Can you work these out from the model? Positions are in its coordinate system, mm. A direction names the side the tool comes from. Round coordinates to 2 decimals unless told otherwise and drop trailing zeros. Loops run counter-clockwise (first coordinate to the right, second up) from the corner with the lowest first, then second, coordinate; pieces in that order, holes last. Notation, with made-up numbers: (-29, 35.5) -> (-11, 35.5) arc R18 cw to (-11, 55.5) -> close; hole circle Ø2 at (-39, 80). An arc over 180 degrees is marked (long way). Write item = value, one per line.
Autodesk Inventor part; units mm, degrees
ref_plane "YZ Plane" through (0, 0, 0) normal (1, 0, 0) x (0, 1, 0)
ref_plane "XZ Plane" through (0, 0, 0) normal (0, 1, 0) x (-1, 0, 0)
ref_plane "XY Plane" through (0, 0, 0) normal (0, 0, 1) x (1, 0, 0)
sketch "Sketch1" plane through (0, 0, 0) normal (0, 1, 0) x (-1, 0, 0)
  line L0 (0, 0) -> (105, 0)
  line L1 (105, 0) -> (105, 30)
  line L2 (105, 30) -> (0, 30)
  line L3 (0, 30) -> (0, 0)
  line L4 (105, 0) -> (65, 0)
  line L5 (65, 0) -> (65, 15)
  line L6 (65, 15) -> (105, 15)
  line L7 (105, 15) -> (105, 0)
  line L8 (0, 15) -> (15, 15)
  line L9 (15, 15) -> (45, 15)
  circle A0 centre (15, 15) radius 4
  circle A1 centre (45, 15) radius 7.5
  dimension "d0" = 105
  dimension "d1" = 30
  dimension "d2" = 40
  dimension "d3" = 15
  dimension "d4" = 15
  dimension "d5" = 30
  dimension "d6" = 8
  dimension "d7" = 15
extrude "Extrusion1" add sketch "Sketch1" along normal blind 55 contours L3 L2 L1 L6 L5 L0
sketch "Sketch2" plane through (-105, 0, 30) normal (0, 0, 1) x (1, 0, 0)
  line L0 (105, 55) -> (81, 55)
  line L1 (81, 55) -> (81, 15)
  line L2 (81, 15) -> (105, 15)
  line L3 (105, 15) -> (105, 55)
  dimension "d10" = 24
  dimension "d11" = 40
extrude "Extrusion2" cut sketch "Sketch2" against normal blind 55
sketch "Sketch3" plane through (-65, 0, 15) normal (0, 0, -1) x (-1, 0, 0)
  line L0 (40, 55) -> (0, 55)
  line L1 (0, 55) -> (0, 40)
  line L2 (0, 40) -> (40, 40)
  line L3 (40, 40) -> (40, 55)
  circle A0 centre (20, 20) radius 4
  point P0 (-65, 0)
  dimension "d15" = 15
  dimension "d16" = 8
extrude "Extrusion3" cut sketch "Sketch3" against normal blind 55
properties part number "X_Top_PullySide_V2" material "Birch"
1. Suppose I cut it at D-D, the plane z = 17.5. List the corners of the cut face in (x, y) for me.
Entries:
outline = (-105, 0) -> (-52.07, 0) -> (-52.07, 55) -> (-65, 55) -> (-65, 40) -> (-105, 40) -> close; (-37.93, 0) -> (-18.12, 0) -> (-18.12, 15) -> (-24, 15) -> (-24, 55) -> (-37.93, 55) -> close; (-11.88, 0) -> (0, 0) -> (0, 15) -> (-11.88, 15) -> close; hole circle Ø8 at (-85, 20)
2. For faces 4 (the cylindrical face through (-82.05, 22.7, 22.4)), 5 (the flat face through (-85, 40, 22)), 6 (the flat face through (-10, 15, 15)), 7 (the cylindrical face through (-52.154, 27.115, 12.747)), 8 (the flat face through (-80, 20, 15)), which set-ups out of +Z, -Z, +X, -X, +Y, -Y let a thin tool reach every point of the face, with its end or its side?
Entries:
face_4 = +Z, -Z
face_5 = +Z, -Z, -X, +Y
face_6 = +Z, -Z, +X, +Y
face_7 = +Y, -Y
face_8 = -Z, -X, +Y, -Y
3. I'm going to push flat-ended pins straight in: pin 1 (4 mm diameter, centred on y = 15, z = 17.5, fed in from +X); pin 2 (9 mm diameter, centred on y = 38, z = 19.5, fed in from +X); pin 3 (7.5 mm diameter, centred on x = -87.5, z = 24, fed in from +Y). Where does each tip first touch, or does it pass through?
Entries:
pin_1 = 0
pin_2 = -24
pin_3 = 40
4. We'd pull the mould along Z, two halves only. Please class faces 1 (the flat face through (-39, 27, 0)), 2 (the cylindrical face through (-11, 7, 15)), 3 (the flat face through (-52, 0, 19)): released by +Z, released by -Z, zero draft, split by the parting line, or undercut.
Entries:
face_1 = released by -Z
face_2 = undercut
face_3 = zero draft
5. Suppose I cut it at C-C, the plane y = 20. List the corners of the cut face in (x, z) for me.
Entries:
outline = (-105, 15) -> (-89, 15) -> (-89, 30) -> (-105, 30) -> close; (-81, 15) -> (-65, 15) -> (-65, 0) -> (-24, 0) -> (-24, 30) -> (-81, 30) -> close; hole circle Ø15 at (-45, 15)
6. Suppose I cut it at B-B, the plane z = 26.5. List the corners of the cut face in (x, y) for me, and give its area (3 significant figures).
Entries:
outline = (-105, 0) -> (0, 0) -> (0, 15) -> (-24, 15) -> (-24, 55) -> (-65, 55) -> (-65, 40) -> (-105, 40) -> close; hole circle Ø8 at (-85, 20)
area = 4,160 mm²
7. Suppose I cut it at A-A, the plane x = -45. List the corners of the cut face in (y, z) for me, and give its area (3 significant figures).
Entries:
outline = (0, 0) -> (55, 0) -> (55, 7.5) -> (0, 7.5) -> close; (0, 22.5) -> (55, 22.5) -> (55, 30) -> (0, 30) -> close
area = 825 mm²
8. I need wall thicknesses on line 1 (Z direction, x = -45, y = 23); line 2 (Z direction, x = -15, y = 7); line 3 (Y direction, x = -85, z = 19.75). Which ranges of each line are inside material? Lowest first, please. Write a range as [from, to].
Entries:
line_1 = [0, 7.5], [22.5, 30]
line_2 = [0, 11], [19, 30]
line_3 = [0, 16], [24, 40]
